```python
from build123d import *

# Parameters (mm, degrees)
SKETCH1_W           = 50.8
SKETCH1_H           = 76.2
SKETCH1_R           = 15.24
SKETCH1_R_2         = 7.62
BOSS_EXTRUDE1_DEPTH = 101.6
CHAMFER1_SIZE       = 6.35


with BuildPart() as part:
    # Sketch1 → Boss-Extrude1 (new body)
    with BuildSketch(Plane.YZ):
        Rectangle(SKETCH1_W, SKETCH1_H)
        with Locations(Location((0, -7.62, 0), (0, 0, 270))):
            Circle(SKETCH1_R, mode=Mode.SUBTRACT)
        with Locations(Location((0, 22.86, 0), (0, 0, 270))):
            Circle(SKETCH1_R_2, mode=Mode.SUBTRACT)
    extrude(amount=BOSS_EXTRUDE1_DEPTH)

    # Chamfer1
    chamfer1_edges = [part.edges().sort_by_distance(p)[0] for p in [
        (50.8, 25.4, 38.1),
        (50.8, 25.4, -38.1),
    ]]
    chamfer(chamfer1_edges, length=CHAMFER1_SIZE)


solid = part.part
```
Could you check a few things on this model? Use its own coordinates, in mm. Round coordinates to 2 decimals unless told otherwise and drop trailing zeros. Loops run counter-clockwise (first coordinate to the right, second up) from the corner with the lowest first, then second, coordinate; pieces in that order, holes last. Notation, with made-up numbers: M 31.5,88 L 53.5,88 A7 cw 53.5,99 Z; hole C 40,-23 d5. An arc over 180 degrees is marked long. Write item = value, one per line.
1. I need wall thicknesses on probe 1 along Y at (x, z) = (54, -7); probe 2 along Z at (x, y) = (20.5, 7); probe 3 along Y at (x, z) = (66, 22.86). Which ranges of each line are inside material? Lowest first, please.
Results below:
probe_1 = -25.4 to -15.23, 15.23 to 25.4
probe_2 = -38.1 to -21.16, 5.92 to 19.85, 25.87 to 38.1
probe_3 = -25.4 to -7.62, 7.62 to 25.4
2. Thinking about a two-plate mould opening in Z: for faces 1 (the face through (50, -3, -38.1)), 2 (the face through (50, -3, 38.1)), 3 (the face through (50.089, 0.335, 30.473)), 4 (the face through (50, 25.4, 0)), which applies, +Z half, -Z half, draft (parallel to the pull), parting line (faces both ways), or undercut?
Results below:
face_1 = -Z half
face_2 = +Z half
face_3 = undercut
face_4 = draft
3. I want a section at C-C, the plane y = 0. Write out the boundary of the cut face in (x, z), and give its area (3 significant figures).
Results below:
outline = M 0,-38.1 L 101.6,-38.1 L 101.6,-22.86 L 0,-22.86 Z; M 0,7.62 L 101.6,7.62 L 101.6,15.24 L 0,15.24 Z; M 0,30.48 L 101.6,30.48 L 101.6,38.1 L 0,38.1 Z
area = 3,100 mm²
4. I want a section at D-D, the plane z = 22.86. Write out the boundary of the cut face in (x, y), and give its area (3 significant figures).
Results below:
outline = M 0,-25.4 L 101.6,-25.4 L 101.6,-7.62 L 0,-7.62 Z; M 0,7.62 L 101.6,7.62 L 101.6,25.4 L 0,25.4 Z
area = 3,610 mm²
5. I want a section at B-B, the plane x = 7. Write out the boundary of the cut face in (y, z).
Results below:
outline = M -25.4,-38.1 L 19.05,-38.1 L 25.4,-31.75 L 25.4,31.75 L 19.05,38.1 L -25.4,38.1 Z; hole C 0,-7.62 d30.48; hole C 0,22.86 d15.24
6. I want a section at A-A, the plane z = -7.62. Write out the boundary of the cut face in (x, y), and give its area (3 significant figures).
Results below:
outline = M 0,-25.4 L 101.6,-25.4 L 101.6,-15.24 L 0,-15.24 Z; M 0,15.24 L 101.6,15.24 L 101.6,25.4 L 0,25.4 Z
area = 2,060 mm²
